Part print with two shaded views. Sizes in mm from the minimum x, y, z corner. A direction names the side the tool comes from. Round coordinates to 2 decimals unless told otherwise and drop trailing zeros. Loops run counter-clockwise (first coordinate to the right, second up) from the corner with the lowest first, then second, coordinate; pieces in that order, holes last.
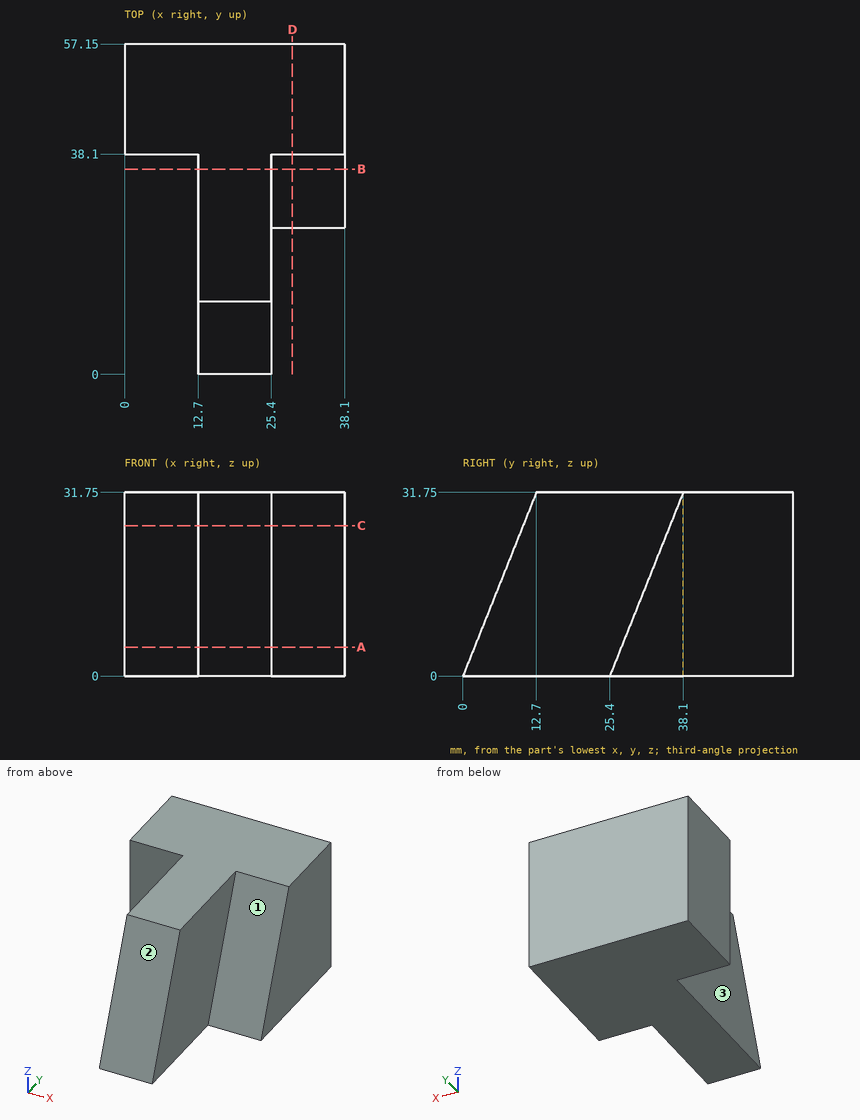
Item 1: Cut at C-C (z = 26). List the corners of the cut face in (x, y).
Verdict:
outline: (0, 38.1) - (12.7, 38.1) - (12.7, 10.4) - (25.4, 10.4) - (25.4, 35.8) - (38.1, 35.8) - (38.1, 57.15) - (0, 57.15) - close
Item 2: Cut at B-B (y = 35.5). List the corners of the cut face in (x, z), plus the area to 3 significant figures.
Verdict:
outline: (12.7, 0) - (38.1, 0) - (38.1, 25.25) - (25.4, 25.25) - (25.4, 31.75) - (12.7, 31.75) - close
area: 724 mm2
Item 3: Flat gauge pins, fed straight in: P1, Ø8, axis at y = 22.5, z = 14.5, coming from the -X side; P2, Ø6.5, axis at x = 4.5, z = 15, coming from the -Y side; P3, Ø9.5, axis at y = 20, z = 21, coming from the +X side. Where does each tip first touch, or does it go through?
Verdict:
P1: stops at x = 12.7
P2: stops at y = 38.1
P3: stops at x = 25.4
Item 4: Wall check: L1, parallel to Y at x = 10, z = 10; L2, parallel to X at y = 6, z = 5.5; L3, parallel to Y at x = 32, z = 27.5. Give the ranges that are in metal, low to high.
Verdict:
L1: y = 38.1 to 57.15
L2: x = 12.7 to 25.4
L3: y = 36.4 to 57.15
Item 5: Cut at D-D (x = 29). List the corners of the cut face in (y, z), plus the area to 3 significant figures.
Verdict:
outline: (25.4, 0) - (57.15, 0) - (57.15, 31.75) - (38.1, 31.75) - close
area: 806 mm2
Item 6: 3-axis set-ups, long thin cutter, end or side, ignore diameter. For the marked faces 1, 2 and 3: which of +Z, -Z, +X, -X, +Y, -Y reach the whole face in a straight line?
Verdict:
face 1: +Z, +X, -Y
face 2: +Z, +X, -X, -Y
face 3: +Z, -Z, -X, -Y
Item 7: Cut at A-A (z = 5). List the corners of the cut face in (x, y), plus the area to 3 significant figures.
Verdict:
outline: (0, 38.1) - (12.7, 38.1) - (12.7, 2) - (25.4, 2) - (25.4, 27.4) - (38.1, 27.4) - (38.1, 57.15) - (0, 57.15) - close
area: 1,320 mm2
